from build123d import *

# Parameters (mm, degrees)
F1_DEPTH = 19.05
F3_DEPTH = 19.05


with BuildPart() as f1:
    # F0 (on Front) → F1 (new body)
    with BuildSketch(Plane.XZ):
        Polygon((-63.5, 0), (0, 0), (-263.9645430735, 457.2), (-327.4645430735, 457.2), align=None)
    extrude(amount=F1_DEPTH)

    # F2 (on face) → F3 (join)
    with BuildSketch(Plane(origin=(0, 0, 0), x_dir=(-1, 0, 0), z_dir=(0, 1, 0))):
        Polygon((130.1731683118, 225.4665412982), (162.2384621855, 281.0052594471), (63.5, 457.2), (0, 457.2), align=None)
        Polygon((161.4879657143, 169.7201351475), (193.5152767914, 225.1930651629), (162.2384621855, 281.0052594471), (130.1731683118, 225.4665412982), align=None)
        Polygon((256.2212291294, 1.0765731137), (319.7121024132, 0), (193.5152767914, 225.1930651629), (161.4879657143, 169.7201351475), align=None)
    extrude(amount=F3_DEPTH)


solid = f1.part
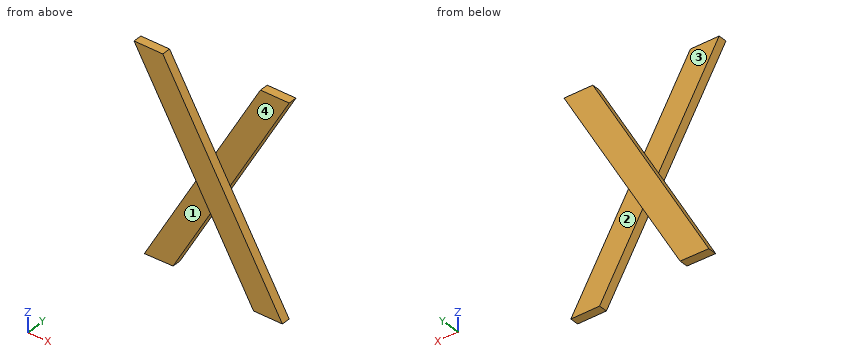
Model file for the job. Use its own axes, mm. Face numbers are marked on the shaded views. A direction names the side the tool comes from. Give positions to 0.01 mm unless a question says otherwise; leave off trailing zeros. Order: outer loops, then holes, each group sorted by start corner. A loop starts at its lowest first (then second) coordinate and runs counter-clockwise, first axis right, second up. Notation, with made-up numbers: M 42.25,82 L 80.25,82 A14 cw 80.25,92 Z; hole C 79,55.25 d6. An arc over 180 degrees is marked long. Put each result on its own line as item: value. Start each with the question number.
(1) Drill centre lines: L1, parallel to Y at x = -308, z = 433.5; L2, parallel to Y at x = -253, z = 93; L3, parallel to X at y = -8, z = 192. Where is each one in solid material? Low to high. Write a range as [from, to].
(2) Pin check, flat tips, straight feed: pin 1 Ø3 at (y, z) = (9.5, 282) entering from -X; pin 2 Ø4 at (y, z) = (5, 181.5) entering from -X; pin 3 Ø10 at (x, y) = (-81, 8) entering from +Z. Stop position of each tip, or through.
(3) Tool access for the marked faces 1, 2, 3 and 4: list every direction of +Z, -Z, +X, -X, +Y, -Y with a clear straight run to the whole face (end or side of a thin tool).
(4) Band-saw the part on C-C on x = -167. Give the cut face in (y, z).
(5) Band-saw the part on D-D on z = 250.5. Give the cut face in (x, y), then the cut area to 3 significant figures.
(6) Band-saw the part on B-B on x = -305.5. Give the cut face in (y, z).
(7) Band-saw the part on A-A on z = 350. Give the cut face in (x, y), then the cut area to 3 significant figures.
Results below:
1. L1: y = [-19.05, 0]
1. L2: y = [0, 19.05]
1. L3: x = [-174.35, -110.85]
2. pin 1: stops at x = -162.52
2. pin 2: stops at x = -219.12
2. pin 3: stops at z = 434.89
3. face 1: -Z, -X, -Y
3. face 2: -Z, +X, +Y
3. face 3: +Z, -X, +Y
3. face 4: +Z, +X, -Y
4. outline: M -19.05,179.27 L 0,179.27 L 0,159.91 L 19.05,159.91 L 19.05,272.51 L 0,272.51 L 0,289.25 L -19.05,289.25 Z
5. outline: M -208.13,-19.05 L -144.63,-19.05 L -144.63,0 L -116.11,0 L -116.11,19.05 L -179.33,19.05 L -179.33,0 L -208.13,0 Z
5. area: 2,410 mm2
6. outline: M -19.05,419.16 L 0,419.16 L 0,457.2 L -19.05,457.2 Z; M 0,0.24 L 19.05,0.24 L 19.05,25.36 L 0,25.36 Z
7. outline: M -265.57,-19.05 L -202.07,-19.05 L -202.07,0 L -265.57,0 Z; M -123.57,0 L -60.22,0 L -60.22,19.05 L -123.57,19.05 Z
7. area: 2,420 mm2
